Geometry: final body of the model. Coordinates: model frame, mm. Coordinates: 2 decimals unless noted, no trailing zeros. Loops run counter-clockwise (first coordinate to the right, second up) from the corner with the lowest first, then second, coordinate; pieces in that order, holes last. Notation, with made-up numbers: (-24, 48.5) - (2, 48.5) arc R13 ccw to (2, 59.5) - close; hole circle Ø6 at (55.25, 14.25). An arc over 180 degrees is marked (long way). Write each question's results on one line, items separated by ' | '. Start each with the question number.
from build123d import *

# Parameters (mm, degrees)
F0_W     = 84.2862705333
F0_H     = 62.5252984464
F1_DEPTH = 38.1
F2_DEPTH = 19.431
F4_DEPTH = 76.2
F5_DEPTH = 50.8
F6_DEPTH = 19.05
F7_R     = 5.08


with BuildPart() as f1:
    # F0 (on Top) → F1 (new body)
    with BuildSketch(Plane.XY):
        with Locations((-0.8938079051, 9.4918403774)):
            Rectangle(F0_W, F0_H)
        Polygon((61.8553981185, 40.7544896007), (41.2493273616, 40.7544896007), (41.2493273616, -21.7708088458), align=None)
        Polygon((-43.0369431717, -21.7708088458), (-43.0369431717, 40.7544896007), (-63.6430233717, 40.7544896007), align=None)
        with BuildLine():
            Line((41.2493273616, -21.7708088458), (-43.0369431717, -21.7708088458))
            ThreePointArc((-43.0369431717, -21.7708088458), (-24.4435818385, -37.0758276989), (-0.8938079051, -42.1121791005))
            ThreePointArc((-0.8938079051, -42.1121791005), (22.5826118494, -36.9238529276), (41.2493273616, -21.7708088458))
        make_face()
    extrude(amount=F1_DEPTH)

    # F2 (add): a face of the model
    f2_faces = [f1.faces().sort_by_distance(p)[0] for p in [
        (-0.8938126266, 40.7544896007, 19.05),
    ]]
    extrude(f2_faces, amount=F2_DEPTH)

    # F3 (on Right) → F4 (join, symmetric)
    with BuildSketch(Plane.YZ):
        with BuildLine():
            add(Edge.make_bspline(
                [(-42.3909127712, 38.0631349981), (-29.9156566507, 46.1025365559), (-0.9292461645, 64.7821826505), (83.4228372852, 77.6600402112), (128.7347014113, 77.0774025905), (150.1817703247, 76.8016278744)],
                knots=[0, 0, 0, 0, 0.2846618796, 0.6614152802, 1, 1, 1, 1], degree=3))
            Line((-42.3909127712, 38.0631349981), (150.1817703247, 38.0631349981))
            Line((150.1817703247, 38.0631349981), (150.1817703247, 76.8016278744))
        make_face()
    extrude(amount=F4_DEPTH, both=True)

    # F5 (cut): a face of the model
    f5_faces = [f1.faces().sort_by_distance(p)[0] for p in [
        (0.4832953146, 74.166117784, 38.0631349981),
    ]]
    extrude(f5_faces, amount=-F5_DEPTH, mode=Mode.SUBTRACT)

    # F6 (cut): a face of the model
    f6_faces = [f1.faces().sort_by_distance(p)[0] for p in [
        (-0.9060877903, 15.8917005053, 0),
    ]]
    extrude(f6_faces, amount=-F6_DEPTH, mode=Mode.SUBTRACT)

    # F7
    f7_edges = [f1.edges().sort_by_distance(p)[0] for p in [
        (-53.339983, 9.49184, 19.05),
        (51.552363, 9.49184, 19.05),
        (51.296645, 8.715914, 63.106757),
        (0, 6.644686, 62.484239),
        (61.855398, 50.46999, 19.05),
        (-63.643023, 50.46999, 19.05),
        (61.855398, 50.453515, 71.874141),
        (-63.643023, 50.453515, 71.874141),
        (-53.105319, 8.779795, 63.12556),
    ]]
    fillet(f7_edges, radius=F7_R)


solid = f1.part
1) Material intervals for line 1 (Z direction, x = 14, y = 28.5); line 2 (Z direction, x = 26.5, y = -1); line 3 (X direction, y = 33, z = 52), sorted ascending. Write a range as [from, to].
2) Section query A-A on z = 28.5. Output: boundary loops of the cut face in (x, y), and give its area (3 significant figures).
3) Pin query (flat end, axial travel): pin 1 Ø3 at (y, z) = (-23, 39) entering from -X; pin 2 Ø6 at (x, z) = (39.5, 49) entering from -Y; pin 3 Ø5 at (x, z) = (44.5, 55.5) entering from -Y. Return the tip coordinate at first contact, or that it passes through.
Returned:
1) line 1: z = [19.05, 68.01] | line 2: z = [19.05, 59.94] | line 3: x = [-61.09, 59.3]
2) outline: (-63.64, 40.75) - (-43.04, -21.77) arc R50.86 ccw to (-0.89, -42.11) arc R52.24 ccw to (41.25, -21.77) - (61.86, 40.75) - (61.86, 60.19) - (-63.64, 60.19) - close | area: 10,200 mm²
3) pin 1: stops at x = -43.13 | pin 2: stops at y = -26.7 | pin 3: stops at y = -12.96
